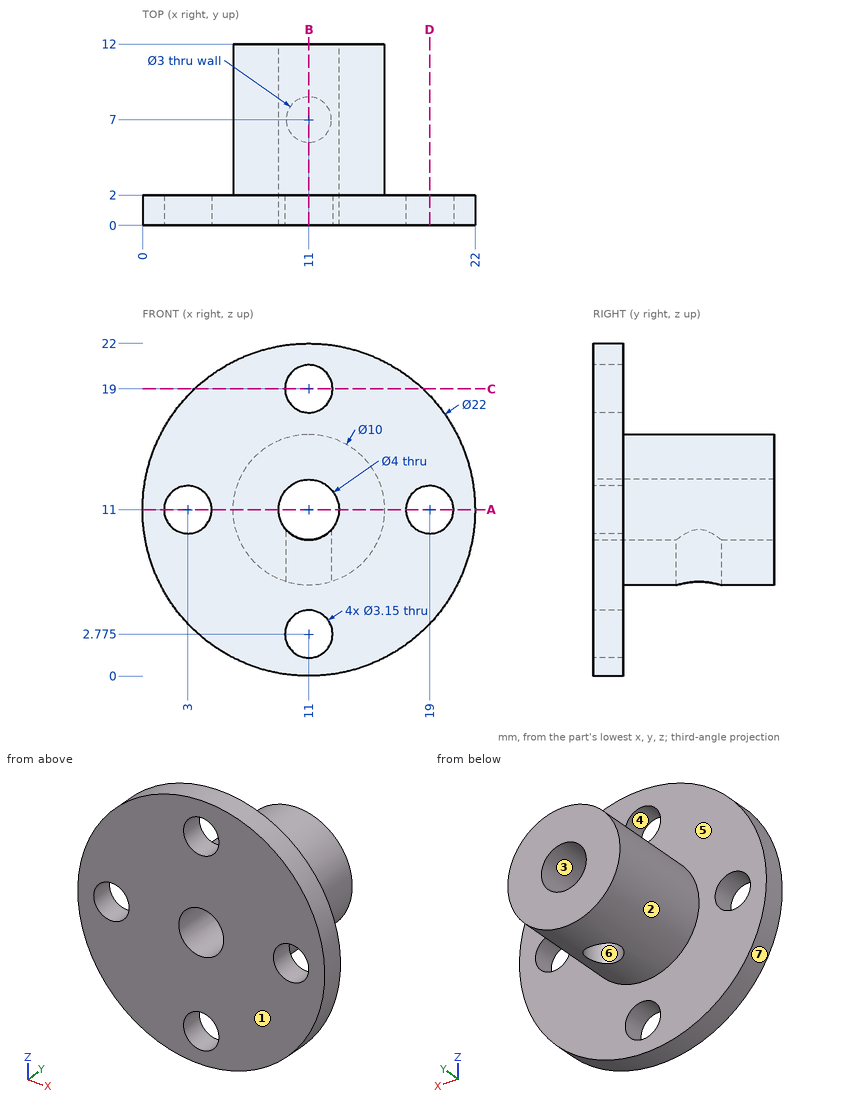
Could you check a few things on this drawing? It's one solid part, dimensions in mm from its lowest x, y, z. A direction names the side the tool comes from. Give positions to 0.01 mm unless a question says otherwise; leave off trailing zeros. Write each loop counter-clockwise with the first axis right and the second up, starting at its lowest first coordinate (ties: lowest second). Pieces come first, ordered by that corner, then holes. Notation, with made-up numbers: (-13, 72) -> (24, 72) arc R18 cw to (24, 102) -> close; hole circle Ø8 at (-23, 33). An arc over 180 degrees is marked (long way). Answer as CSV lines item,"result". Start each with the question number.
(1) Please list where these lines run through material, in increasing order: line 1 (X direction, y = 1, z = 11) (3 decimals); line 2 (Z direction, x = 11, y = 3.5); line 3 (Z direction, x = 9.75, y = 1).
(2) If we section it at D-D, the plane x = 19: Write out the boundary of the cut face in (y, z) (3 decimals), and give its area (3 significant figures).
(3) If we section it at A-A, the plane z = 11: Write out the boundary of the cut face in (x, y) (3 decimals).
(4) I'm going to push flat-ended pins straight in: pin 1 Ø3 at (x, z) = (11, 2.77) entering from +Y; pin 2 Ø2 at (x, y) = (7.5, 10.5) entering from -Z; pin 3 Ø2 at (x, z) = (18.5, 19.5) entering from +Y; pin 4 Ø2 at (x, y) = (12.5, 3.5) entering from -Z (3 decimals). Where does each tip first touch, or does it pass through?
(5) If we mould it in two halves opening along Z, with no side actions, what happens to the marked faces 1, 2, 3 and 4? For each: +Z half, -Z half, draft (parallel to the pull), parting line (faces both ways), or undercut.
(6) If we section it at B-B, the plane x = 11: Write out the boundary of the cut face in (y, z) (3 decimals), and give its area (3 significant figures).
(7) If we section it at C-C, the plane z = 19: Write out the boundary of the cut face in (x, y) (3 decimals).
(8) Which directions (+Z, -Z, +X, -X, +Y, -Y) give clear straight access to the entire face, cutting with the end or side of a thin tool? Please do the marked faces 5, 6 and 7.
Answer list:
1,line 1,"0 to 1.425, 4.575 to 9, 13 to 17.425, 20.575 to 22"
1,line 2,"6 to 9, 13 to 16"
1,line 3,"0.07 to 1.82, 3.73 to 9.44, 12.56 to 18.04, 19.96 to 21.93"
2,outline,"(0, 3.45) -> (2, 3.45) -> (2, 9.425) -> (0, 9.425) -> close; (0, 12.575) -> (2, 12.575) -> (2, 18.55) -> (0, 18.55) -> close"
2,area,"23.9 mm^2"
3,outline,"(0, 0) -> (1.425, 0) -> (1.425, 2) -> (0, 2) -> close; (4.575, 0) -> (9, 0) -> (9, 12) -> (6, 12) -> (6, 2) -> (4.575, 2) -> close; (13, 0) -> (17.425, 0) -> (17.425, 2) -> (16, 2) -> (16, 12) -> (13, 12) -> close; (20.575, 0) -> (22, 0) -> (22, 2) -> (20.575, 2) -> close"
4,pin 1,"through"
4,pin 2,"z = 6.67"
4,pin 3,"y = 2"
4,pin 4,"z = 6.025"
5,face 1,"draft"
5,face 2,"parting line"
5,face 3,"undercut"
5,face 4,"undercut"
6,outline,"(0, 0) -> (2, 0) -> (2, 1.2) -> (0, 1.2) -> close; (0, 4.35) -> (2, 4.35) -> (2, 6) -> (5.5, 6) -> (5.5, 9) -> (0, 9) -> close; (0, 13) -> (12, 13) -> (12, 16) -> (2, 16) -> (2, 17.425) -> (0, 17.425) -> close; (0, 20.575) -> (2, 20.575) -> (2, 22) -> (0, 22) -> close; (8.5, 6) -> (12, 6) -> (12, 9) -> (8.5, 9) -> close"
6,area,"74.4 mm^2"
7,outline,"(3.45, 0) -> (9.425, 0) -> (9.425, 2) -> (3.45, 2) -> close; (12.575, 0) -> (18.55, 0) -> (18.55, 2) -> (12.575, 2) -> close"
8,face 5,"+Y"
8,face 6,"-Z"
8,face 7,"+Y, -Y"
